Model file for the job. Use its own axes, mm. Give positions to 0.01 mm unless a question says otherwise; leave off trailing zeros. Write each loop counter-clockwise with the first axis right and the second up, starting at its lowest first coordinate (ties: lowest second). Pieces come first, ordered by that corner, then holes.
```python
from build123d import *

# Parameters (mm, degrees)
PAD_DEPTH       = 10.6
PAD005_DEPTH    = 2
FILLET_R        = 4
FILLET008_R     = 7
CHAMFER_ANGLE   = 30
CHAMFER_SIZE    = 6
FILLET009_R     = 1
FILLET010_R     = 1.2
CHAMFER004_SIZE = 0.2
SKETCH015_R     = 1.25
HOLE004_DEPTH   = 3
HOLE004_TIPS_R  = 1.25


with BuildPart() as part:
    # Sketch → Pad (new body)
    with BuildSketch(Plane.XY):
        Polygon((-152.075, 56.825), (152.075, 56.825), (152.075, -37.775), (113.975, -37.775), (104.45, -56.825), (-123.5, -56.825), (-133.025, -37.775), (-152.075, -37.775), align=None)
        Polygon((-143.075, 47.825), (143.075, 47.825), (143.075, -28.775), (100.2125, -28.775), (100.2125, -47.825), (-119.2625, -47.825), (-119.2625, -28.775), (-143.075, -28.775), align=None, mode=Mode.SUBTRACT)
    extrude(amount=PAD_DEPTH)

    # Sketch011 (on Face17 of Pad) → Pad005 (join)
    with BuildSketch(Plane(origin=(0, 0, 0), x_dir=(1, 0, 0), z_dir=(0, 0, -1))):
        with BuildLine():
            ThreePointArc((16.752533, -47.408333), (14.2875, -45.325), (11.822467, -47.408333))
            ThreePointArc((11.32946, -47.825), (11.652209, -47.706881), (11.822467, -47.408333))
            Line((11.32946, -47.825), (17.24554, -47.825))
            ThreePointArc((16.752533, -47.408333), (16.922791, -47.706881), (17.24554, -47.825))
        make_face()
        with BuildLine():
            ThreePointArc((112.002533, -47.408333), (109.5375, -45.325), (107.072467, -47.408333))
            ThreePointArc((106.57946, -47.825), (106.902209, -47.706881), (107.072467, -47.408333))
            Line((106.57946, -47.825), (112.49554, -47.825))
            ThreePointArc((112.002533, -47.408333), (112.172791, -47.706881), (112.49554, -47.825))
        make_face()
        with BuildLine():
            ThreePointArc((-97.547467, -47.408333), (-100.0125, -45.325), (-102.477533, -47.408333))
            ThreePointArc((-102.97054, -47.825), (-102.647791, -47.706881), (-102.477533, -47.408333))
            Line((-102.97054, -47.825), (-97.05446, -47.825))
            ThreePointArc((-97.547467, -47.408333), (-97.377209, -47.706881), (-97.05446, -47.825))
        make_face()
        with BuildLine():
            ThreePointArc((73.734967, 47.408333), (76.2, 45.325), (78.665033, 47.408333))
            ThreePointArc((79.15804, 47.825), (78.835291, 47.706881), (78.665033, 47.408333))
            Line((73.24196, 47.825), (79.15804, 47.825))
            ThreePointArc((73.734967, 47.408333), (73.564709, 47.706881), (73.24196, 47.825))
        make_face()
        with BuildLine():
            ThreePointArc((-97.715033, 47.408333), (-95.25, 45.325), (-92.784967, 47.408333))
            ThreePointArc((-92.29196, 47.825), (-92.614709, 47.706881), (-92.784967, 47.408333))
            Line((-98.20804, 47.825), (-92.29196, 47.825))
            ThreePointArc((-97.715033, 47.408333), (-97.885291, 47.706881), (-98.20804, 47.825))
        make_face()
    extrude(amount=-PAD005_DEPTH)

    # Fillet
    fillet_edges = [part.edges().sort_by_distance(p)[0] for p in [
        (113.975, -37.775, 5.3),
        (-133.025, -37.775, 5.3),
    ]]
    fillet(fillet_edges, radius=FILLET_R)

    # Fillet008
    fillet008_edges = [part.edges().sort_by_distance(p)[0] for p in [
        (-152.075, -37.775, 5.3),
        (-123.5, -56.825, 5.3),
        (104.45, -56.825, 5.3),
        (152.075, -37.775, 5.3),
        (152.075, 56.825, 5.3),
        (-152.075, 56.825, 5.3),
    ]]
    fillet(fillet008_edges, radius=FILLET008_R)

    # Chamfer
    chamfer_edges = [part.edges().sort_by_distance(p)[0] for p in [
        (-9.525, -56.825, 10.6),
    ]]
    chamfer_side = part.faces().sort_by_distance((130.761068, -34.528101, 10.6))[0]
    chamfer(chamfer_edges, length=CHAMFER_SIZE, angle=CHAMFER_ANGLE, reference=chamfer_side)

    # Fillet009
    fillet009_edges = [part.edges().sort_by_distance(p)[0] for p in [
        (100.2125, -47.825, 5.3),
        (143.075, -28.775, 5.3),
        (143.075, 47.825, 5.3),
        (-143.075, 47.825, 5.3),
        (-143.075, -28.775, 5.3),
        (-119.2625, -47.825, 5.3),
    ]]
    fillet(fillet009_edges, radius=FILLET009_R)

    # Fillet010
    fillet010_edges = [part.edges().sort_by_distance(p)[0] for p in [
        (100.2125, -28.775, 5.3),
        (-119.2625, -28.775, 5.3),
    ]]
    fillet(fillet010_edges, radius=FILLET010_R)

    # Chamfer004
    chamfer004_edges = [part.edges().sort_by_distance(p)[0] for p in [
        (121.74375, -28.775, 10.6),
        (121.74375, -28.775, 0),
        (152.075, 9.525, 0),
    ]]
    chamfer(chamfer004_edges, length=CHAMFER004_SIZE)

    # Sketch015 (on Face118 of Chamfer004) → Hole004 (cut)
    with BuildSketch(Plane(origin=(0, 0, 0), x_dir=(1, 0, 0), z_dir=(0, 0, -1))):
        with Locations((-95.25, 52.325)):
            Circle(SKETCH015_R)
        with Locations((95.25, 52.325)):
            Circle(SKETCH015_R)
        with Locations((147.575, 19.05)):
            Circle(SKETCH015_R)
        with Locations((-147.575, 19.05)):
            Circle(SKETCH015_R)
        with Locations((-147.575, -52.325)):
            Circle(SKETCH015_R)
        with Locations((147.575, -52.325)):
            Circle(SKETCH015_R)
        with Locations((-19.05, -52.325)):
            Circle(SKETCH015_R)
        with Locations((19.05, -52.325)):
            Circle(SKETCH015_R)
    extrude(amount=-HOLE004_DEPTH, mode=Mode.SUBTRACT)

    # Hole004 tips → Hole004 tip 1 section 0
    with BuildSketch(Plane(origin=(0, 0, 3), x_dir=(1, 0, 0), z_dir=(0, 0, -1)), mode=Mode.PRIVATE) as hole004_tip_1_s0:
        with Locations((-95.25, 52.325)):
            Circle(HOLE004_TIPS_R)
    loft([hole004_tip_1_s0.sketch, Vertex(-95.25, -52.325, 3.751076)], mode=Mode.SUBTRACT)

    # Hole004 tips → Hole004 tip 2 section 0
    with BuildSketch(Plane(origin=(0, 0, 3), x_dir=(1, 0, 0), z_dir=(0, 0, -1)), mode=Mode.PRIVATE) as hole004_tip_2_s0:
        with Locations((95.25, 52.325)):
            Circle(HOLE004_TIPS_R)
    loft([hole004_tip_2_s0.sketch, Vertex(95.25, -52.325, 3.751076)], mode=Mode.SUBTRACT)

    # Hole004 tips → Hole004 tip 3 section 0
    with BuildSketch(Plane(origin=(0, 0, 3), x_dir=(1, 0, 0), z_dir=(0, 0, -1)), mode=Mode.PRIVATE) as hole004_tip_3_s0:
        with Locations((147.575, 19.05)):
            Circle(HOLE004_TIPS_R)
    loft([hole004_tip_3_s0.sketch, Vertex(147.575, -19.05, 3.751076)], mode=Mode.SUBTRACT)

    # Hole004 tips → Hole004 tip 4 section 0
    with BuildSketch(Plane(origin=(0, 0, 3), x_dir=(1, 0, 0), z_dir=(0, 0, -1)), mode=Mode.PRIVATE) as hole004_tip_4_s0:
        with Locations((-147.575, 19.05)):
            Circle(HOLE004_TIPS_R)
    loft([hole004_tip_4_s0.sketch, Vertex(-147.575, -19.05, 3.751076)], mode=Mode.SUBTRACT)

    # Hole004 tips → Hole004 tip 5 section 0
    with BuildSketch(Plane(origin=(0, 0, 3), x_dir=(1, 0, 0), z_dir=(0, 0, -1)), mode=Mode.PRIVATE) as hole004_tip_5_s0:
        with Locations((-147.575, -52.325)):
            Circle(HOLE004_TIPS_R)
    loft([hole004_tip_5_s0.sketch, Vertex(-147.575, 52.325, 3.751076)], mode=Mode.SUBTRACT)

    # Hole004 tips → Hole004 tip 6 section 0
    with BuildSketch(Plane(origin=(0, 0, 3), x_dir=(1, 0, 0), z_dir=(0, 0, -1)), mode=Mode.PRIVATE) as hole004_tip_6_s0:
        with Locations((147.575, -52.325)):
            Circle(HOLE004_TIPS_R)
    loft([hole004_tip_6_s0.sketch, Vertex(147.575, 52.325, 3.751076)], mode=Mode.SUBTRACT)

    # Hole004 tips → Hole004 tip 7 section 0
    with BuildSketch(Plane(origin=(0, 0, 3), x_dir=(1, 0, 0), z_dir=(0, 0, -1)), mode=Mode.PRIVATE) as hole004_tip_7_s0:
        with Locations((-19.05, -52.325)):
            Circle(HOLE004_TIPS_R)
    loft([hole004_tip_7_s0.sketch, Vertex(-19.05, 52.325, 3.751076)], mode=Mode.SUBTRACT)

    # Hole004 tips → Hole004 tip 8 section 0
    with BuildSketch(Plane(origin=(0, 0, 3), x_dir=(1, 0, 0), z_dir=(0, 0, -1)), mode=Mode.PRIVATE) as hole004_tip_8_s0:
        with Locations((19.05, -52.325)):
            Circle(HOLE004_TIPS_R)
    loft([hole004_tip_8_s0.sketch, Vertex(19.05, 52.325, 3.751076)], mode=Mode.SUBTRACT)


solid = part.part
```
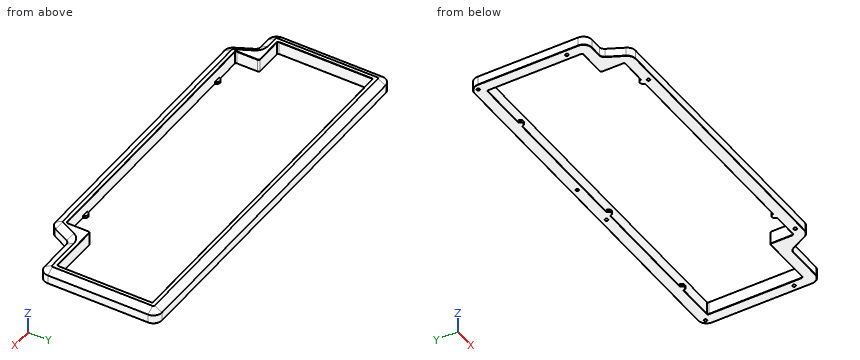
1. Probe probe 1 along Y at (x, z) = (19.05, 2) (3 decimals); probe 2 along X at (y, z) = (-19.05, 1.45) (3 decimals); probe 3 along Y at (x, z) = (99, 2.25) (3 decimals). List the from-to ranges inside material, lowest first.
Calculated:
probe 1: y = -56.825 to -47.825, 47.825 to 51.075, 53.575 to 56.825
probe 2: x = -152.075 to -148.825, -146.325 to -143.075, 143.075 to 146.325, 148.825 to 152.075
probe 3: y = -56.825 to -47.825, 47.825 to 56.825
2. Pin check, flat tips, straight feed: P1, Ø2, axis at x = -147.575, y = 52.325, coming from the -Z side; P2, Ø1.5, axis at x = 95.25, y = -52.325, coming from the +Z side; P3, Ø2, axis at x = -138, z = 4, coming from the -Y side (3 decimals). Stop position of each tip, or through.
Calculated:
P1: stops at z = 3.15
P2: stops at z = 10.17
P3: stops at y = -37.775
3. Slice it at B-B, the plane y = 3. Write the cut outline in (x, z) (3 decimals), and give its area (3 significant figures).
Calculated:
outline: (-152.075, 0.2) - (-151.875, 0) - (-143.275, 0) - (-143.075, 0.2) - (-143.075, 10.4) - (-143.275, 10.6) - (-146.075, 10.6) - (-152.075, 7.136) - close; (143.075, 0.2) - (143.275, 0) - (151.875, 0) - (152.075, 0.2) - (152.075, 7.136) - (146.075, 10.6) - (143.275, 10.6) - (143.075, 10.4) - close
area: 170 mm2
4. Slice it at A-A, the plane x = 68.5. Write the cut outline in (y, z) (3 decimals), and give its area (3 significant figures).
Calculated:
outline: (-56.825, 0.2) - (-56.625, 0) - (-48.025, 0) - (-47.825, 0.2) - (-47.825, 10.4) - (-48.025, 10.6) - (-50.825, 10.6) - (-56.825, 7.136) - close; (47.825, 0.2) - (48.025, 0) - (56.625, 0) - (56.825, 0.2) - (56.825, 7.136) - (50.825, 10.6) - (48.025, 10.6) - (47.825, 10.4) - close
area: 170 mm2
